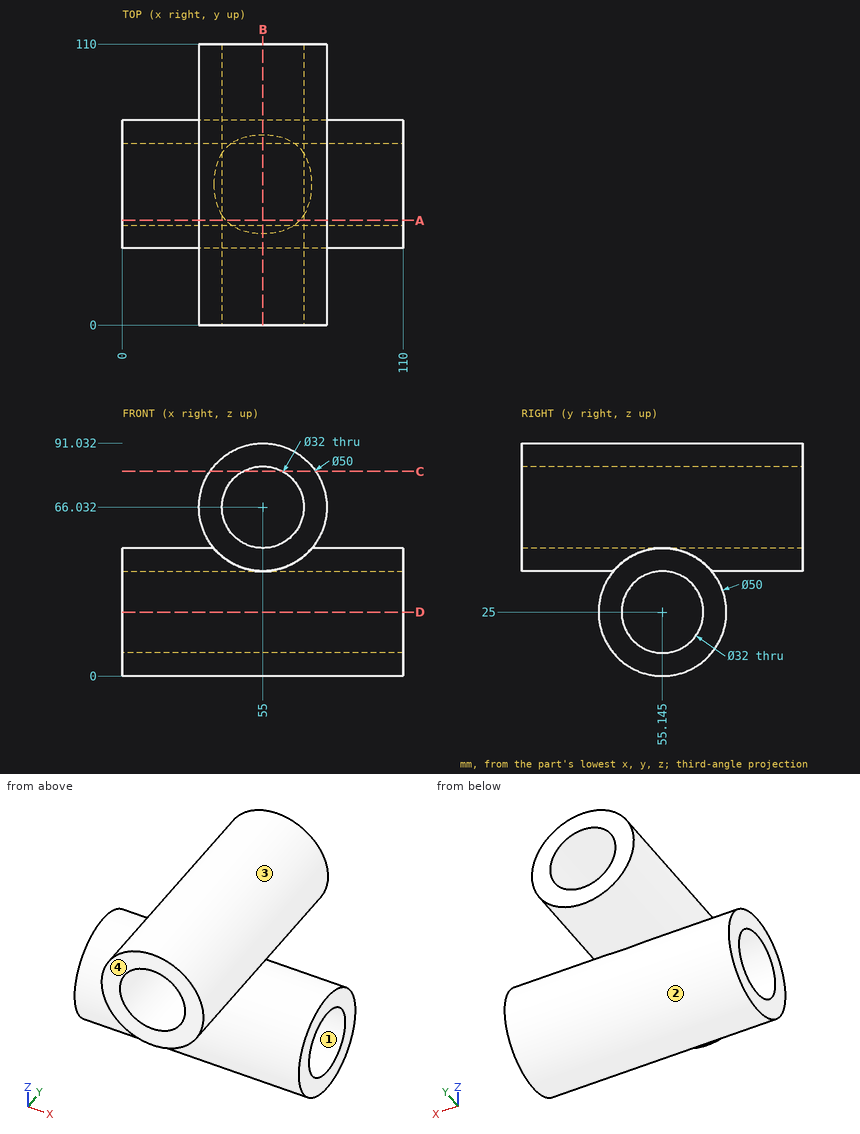
Drawing for the job (mm, zero at the part's lowest x, y, z). A direction names the side the tool comes from. Coordinates: 2 decimals unless noted, no trailing zeros. Order: outer loops, then holes, each group sorted by start corner. A loop starts at its lowest first (then second) coordinate and runs counter-clockwise, first axis right, second up.
Item 1: Band-saw the part on B-B on x = 55. List the corners of the cut face in (y, z) (1 decimal).
Check sheet entries:
outline: (0, 41) - (36, 41) arc R25 ccw (long way) to (74.3, 41) - (110, 41) - (110, 50) - (0, 50) - close; (0, 82) - (110, 82) - (110, 91) - (0, 91) - close; hole circle Ø32 at (55.1, 25)
Item 2: 3-axis set-ups, long thin cutter, end or side, ignore diameter. For the marked faces 1 and 2: which of +Z, -Z, +X, -X, +Y, -Y reach the whole face in a straight line?
Check sheet entries:
face 1: +X, -X
face 2: none
Item 3: Pin check, flat tips, straight feed: pin 1 Ø1.5 at (y, z) = (28.5, 18) entering from -X (3 decimals); pin 2 Ø1 at (y, z) = (79.5, 77.5) entering from +X (1 decimal); pin 3 Ø1 at (x, y) = (68, 18.5) entering from -Z; pin 4 Ø6 at (x, z) = (60, 16.5) entering from -Y. Stop position of each tip, or through.
Check sheet entries:
pin 1: passes through
pin 2: stops at x = 77.5
pin 3: stops at z = 44.38
pin 4: stops at y = 30.76
Item 4: Band-saw the part on A-A on y = 41. List the corners of the cut face in (x, z) (1 decimal).
Check sheet entries:
outline: (0, 4.4) - (110, 4.4) - (110, 17.5) - (0, 17.5) - close; (0, 32.5) - (110, 32.5) - (110, 45.6) - (69.4, 45.6) arc R25 ccw (long way) to (40.6, 45.6) - (0, 45.6) - close; hole circle Ø32 at (55, 66)
Item 5: Band-saw the part on C-C on z = 80. List the corners of the cut face in (x, y).
Check sheet entries:
outline: (34.27, 0) - (47.2, 0) - (47.2, 110) - (34.27, 110) - close; (62.8, 0) - (75.73, 0) - (75.73, 110) - (62.8, 110) - close
Item 6: Two-plate mould, pull along Z, no slides. Class the marked faces 3 and 4: +Z half, -Z half, draft (parallel to the pull), parting line (faces both ways), or undercut.
Check sheet entries:
face 3: undercut
face 4: draft
Item 7: Drill centre lines: L1, parallel to Z at x = 76, y = 63.5 (1 decimal); L2, parallel to Y at x = 41.5, z = 25 (1 decimal); L3, parallel to Z at x = 61, y = 54 (1 decimal). Where is each one in solid material? Low to high.
Check sheet entries:
L1: z = 1.4 to 11.4, 38.6 to 48.6, 52.5 to 79.6
L2: y = 30.1 to 39.1, 71.1 to 80.1
L3: z = 0 to 9, 41 to 51.2, 80.9 to 90.3
Item 8: Band-saw the part on D-D on z = 25. List the corners of the cut face in (x, y) (1 decimal).
Check sheet entries:
outline: (0, 30.1) - (110, 30.1) - (110, 39.1) - (0, 39.1) - close; (0, 71.1) - (110, 71.1) - (110, 80.1) - (0, 80.1) - close
